from build123d import *

# Parameters (mm, degrees)
F1_DEPTH = 15
F2_R     = 1


with BuildPart() as f1:
    # F0 (on Top) → F1 (new body)
    with BuildSketch(Plane.XY):
        Polygon((-40.153805, 40), (-40.153805, 0), (-33.126801, 0), (-33.126801, 29.933507), (-23.060559, 0), (-10.49746, 0), (-10.49746, 40), (-18.119976, 40), (-18.119976, 9.805305), (-28.274053, 40), align=None)
    extrude(amount=F1_DEPTH)

    # F2
    f2_edges = [f1.edges().sort_by_distance(p)[0] for p in [
        (-23.197014, 24.902652, 15),
        (-34.213929, 40, 15),
        (-40.153805, 20, 15),
        (-36.640303, 0, 15),
        (-33.126801, 14.966753, 15),
        (-28.09368, 14.966753, 15),
        (-16.779009, 0, 15),
        (-10.49746, 20, 15),
        (-14.308718, 40, 15),
        (-18.119976, 24.902652, 15),
        (-23.197014, 24.902652, 0),
        (-34.213929, 40, 0),
        (-40.153805, 20, 0),
        (-36.640303, 0, 0),
        (-33.126801, 14.966753, 0),
        (-28.09368, 14.966753, 0),
        (-16.779009, 0, 0),
        (-10.49746, 20, 0),
        (-14.308718, 40, 0),
        (-18.119976, 24.902652, 0),
        (-23.060559, 0, 7.5),
        (-10.49746, 0, 7.5),
        (-40.153805, 0, 7.5),
        (-33.126801, 0, 7.5),
        (-28.274053, 40, 7.5),
        (-40.153805, 40, 7.5),
        (-10.49746, 40, 7.5),
        (-18.119976, 40, 7.5),
        (-33.126801, 29.933507, 7.5),
        (-18.119976, 9.805305, 7.5),
    ]]
    fillet(f2_edges, radius=F2_R)


solid = f1.part
Here's how the part is built. I have some questions about the finished solid (model axes, mm). A direction names the side the tool comes from. Coordinates: 2 decimals unless noted, no trailing zeros. Order: outer loops, then holes, each group sorted by start corner. A loop starts at its lowest first (then second) coordinate and runs counter-clockwise, first axis right, second up. Notation, with made-up numbers: (5.5, 40.25) - (48.5, 40.25) arc R18 cw to (48.5, 45.25) - close; hole circle Ø11 at (62, 33.5). An arc over 180 degrees is marked (long way). Use CSV: the item, a comma, the result in double quotes. Start each with the question number.
1. If we mould it in two halves opening along X, with no side actions, what happens to faces 1 (the face through (-16.844, 0.285, 0.301)), 2 (the face through (-10.798, 0.285, 7.591)), 3 (the face through (-17.835, 27.297, 14.699))? For each: +X half, -X half, draft (parallel to the pull), parting line (faces both ways), or undercut.
2. For faces 4 (the face through (-26.91, 12.34, 14.7)), 5 (the face through (-26.91, 12.34, 0.3)), 6 (the face through (-22.93, 0.19, 7.59)), 7 (the face through (-28.402, 39.807, 7.591)), which set-ups out of +Z, -Z, +X, -X, +Y, -Y let a thin tool reach every point of the face, with its end or its side?
3. Suppose I cut it at A-A on z = 10.75. List the corners of the cut face in (x, y) for me, then the cut area to 3 significant figures.
4. Please list where these lines run through material, in increasing order: line 1 (X direction, y = 22.5, z = 14.25); line 2 (X direction, y = 19, z = 2.5); line 3 (X direction, y = 35.5, z = 3). Write a range as from..to.
5. Suppose I cut it at B-B on y = 22. Give the number of separate pieces and of enclosed holes in the cut face, then the cut area to 3 significant figures.
Output:
1,face 1,"draft"
1,face 2,"+X half"
1,face 3,"undercut"
2,face 4,"+Z, -Y"
2,face 5,"-Z, -Y"
2,face 6,"+Z, -Z, -Y"
2,face 7,"+Z, -Z, +Y"
3,outline,"(-40.15, 1) arc R1 ccw to (-39.15, 0) - (-34.13, 0) arc R1 ccw to (-33.13, 1) - (-33.13, 23.82) arc R1 cw to (-31.18, 24.14) - (-23.29, 0.68) arc R1 ccw to (-22.34, 0) - (-11.5, 0) arc R1 ccw to (-10.5, 1) - (-10.5, 39) arc R1 ccw to (-11.5, 40) - (-17.12, 40) arc R1 ccw to (-18.12, 39) - (-18.12, 15.92) arc R1 cw to (-20.07, 15.6) - (-28.04, 39.32) arc R1 ccw to (-28.99, 40) - (-39.15, 40) arc R1 ccw to (-40.15, 39) - close"
3,area,"890 mm2"
4,line 1,"x = -40.12..-33.16, -30.59..-22.42, -18.09..-10.53"
4,line 2,"x = -40.15..-33.13, -29.45..-21.21, -18.12..-10.5"
4,line 3,"x = -40.15..-26.76, -18.12..-10.5"
5,separate pieces,"3"
5,enclosed holes,"0"
5,area,"341 mm2"
